Source: three-view drawing plus pictorial views. Frame: mm from the lowest corner of the part. Round coordinates to 2 decimals unless told otherwise and drop trailing zeros. Write each loop counter-clockwise with the first axis right and the second up, starting at its lowest first coordinate (ties: lowest second). Pieces come first, ordered by that corner, then holes. Notation, with made-up numbers: M 71,-21.5 L 129,-21.5 A19 cw 129,3.5 Z; hole C 34,-20.5 d4. An arc over 180 degrees is marked long. Put each result on its own line as item: value. Start each with the question number.
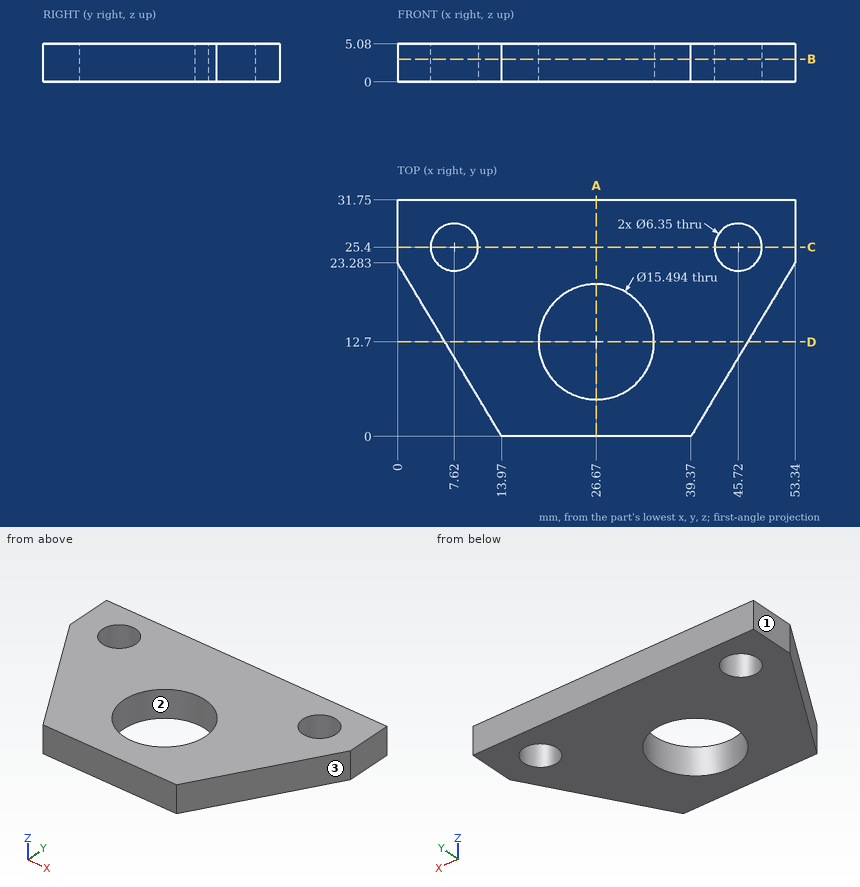
(1) Contact query for flat-ended pins moving along their axis: P1, Ø1.5, axis at y = 21.5, z = 1, coming from the +X side; P2, Ø3, axis at y = 20, z = 4.5, coming from the -X side; P3, Ø1.5, axis at y = 9, z = 1.5, coming from the -X side; P4, Ø12.5, axis at x = 26.67, y = 12.7, coming from the +Z side. Output: stop coordinate, or through.
(2) Section query A-A (x = 26.67). Return loops of the section in (y, z).
(3) Section query C-C (y = 25.4). Return loops of the section in (x, z) (1 decimal).
(4) Pull-direction query (Y, two-part tool) for the marked faces 1, 2 and 3; classes: +Y half, -Y half, draft (parallel to the pull), parting line (faces both ways), or undercut.
(5) Section query B-B (z = 3.05). Count the separate pieces of the cut face and the enclosed holes in it, and give its area (3 significant figures).
(6) Section query D-D (y = 12.7). Return loops of the section in (x, z).
(7) Ray query, line 1 along Y through (x, z) = (26.67, 2.45); line 2 along X through (y, z) = (27, 2.2); line 3 along X through (y, z) = (26.5, 0.4). Return the intervals inside material, ascending.
Entries:
1. P1: x = 52.72
1. P2: x = 1.07
1. P3: x = 8.12
1. P4: through
2. outline: M 0,0 L 4.95,0 L 4.95,5.08 L 0,5.08 Z; M 20.45,0 L 31.75,0 L 31.75,5.08 L 20.45,5.08 Z
3. outline: M 0,0 L 4.4,0 L 4.4,5.1 L 0,5.1 Z; M 10.8,0 L 42.5,0 L 42.5,5.1 L 10.8,5.1 Z; M 48.9,0 L 53.3,0 L 53.3,5.1 L 48.9,5.1 Z
4. face 1: draft
4. face 2: undercut
4. face 3: -Y half
5. separate pieces: 1
5. enclosed holes: 3
5. area: 1,120 mm2
6. outline: M 6.35,0 L 18.92,0 L 18.92,5.08 L 6.35,5.08 Z; M 34.42,0 L 46.99,0 L 46.99,5.08 L 34.42,5.08 Z
7. line 1: 0 to 4.95, 20.45 to 31.75
7. line 2: 0 to 4.88, 10.36 to 42.98, 48.46 to 53.34
7. line 3: 0 to 4.64, 10.6 to 42.74, 48.7 to 53.34
